Here's how the part is built. I have some questions about the finished solid (model axes, mm). Coordinates: 2 decimals unless noted, no trailing zeros. Write each loop counter-clockwise with the first axis right and the second up, starting at its lowest first coordinate (ties: lowest second). Pieces come first, ordered by that corner, then holes.
(1) Imagine slicing it at C-C, the plane y = 15. List the corners of the cut face in (x, z) for me, plus the area to 3 significant figures.
(2) Please list where these lines run through material, in increasing order: probe 1 along Y at (x, z) = (13, -1.2); probe 2 along Y at (x, z) = (128.5, -2.6); probe 3 along X at (y, z) = (39, -2.25).
(3) Imagine slicing it at A-A, the plane y = -23. List the corners of the cut face in (x, z) for me.
(4) Imagine slicing it at B-B, the plane x = 30. List the corners of the cut face in (y, z) for me, plus the area to 3 significant figures.
(5) Imagine slicing it at D-D, the plane z = -1.85. State how many separate pieces and enclosed holes the cut face has, plus the area to 3 significant figures.
```python
from build123d import *

# Parameters (mm, degrees)
SKETCH_1_W             = 270
SKETCH_1_H             = 150
SM_BASE_FLANGE_1_DEPTH = 4
FILLET_1_R             = 1
SKETCH_2_R             = 1.5
CUT_EXTRUDE_1_DEPTH    = 10
SKETCH_3_R             = 1.5
CUT_EXTRUDE_2_DEPTH    = 10
SKETCH_4_W             = 47
SKETCH_4_H             = 90
CUT_EXTRUDE_3_DEPTH    = 10
SKETCH_5_W             = 57
SKETCH_5_H             = 50
CUT_EXTRUDE_4_DEPTH    = 10
SKETCH_6_W             = 14
SKETCH_6_H             = 36.5
CUT_EXTRUDE_5_DEPTH    = 10


# Sheet-metal steps are written as plain solids
with BuildPart() as part:
    # Sketch 1 → 基体-法兰1 (new body)
    with BuildSketch(Plane.XY):
        Rectangle(SKETCH_1_W, SKETCH_1_H)
    extrude(amount=-SM_BASE_FLANGE_1_DEPTH)

    # 圆角1
    fillet_1_edges = [part.edges().sort_by_distance(p)[0] for p in [
        (135, -75, -2),
        (-135, -75, -2),
        (-135, 75, -2),
        (135, 75, -2),
    ]]
    fillet(fillet_1_edges, radius=FILLET_1_R)

    # Sketch 2 → 切除-拉伸1 (cut)
    with BuildSketch(Plane(origin=(0, 0, -4), x_dir=(-1, 0, 0), z_dir=(0, 0, -1))):
        with Locations((-13, -67.5)):
            Circle(SKETCH_2_R)
        with Locations((-13, -57.5)):
            Circle(SKETCH_2_R)
        with Locations((13, -57.5)):
            Circle(SKETCH_2_R)
        with Locations((13, -67.5)):
            Circle(SKETCH_2_R)
    extrude(amount=-CUT_EXTRUDE_1_DEPTH, mode=Mode.SUBTRACT)

    # 草图3 → 切除-拉伸2 (cut)
    with BuildSketch(Plane(origin=(0, 0, -4), x_dir=(-1, 0, 0), z_dir=(0, 0, -1))):
        with Locations((-128.5, 58)):
            Circle(SKETCH_3_R)
        with Locations((-128.5, 32)):
            Circle(SKETCH_3_R)
        with Locations((-118.5, 58)):
            Circle(SKETCH_3_R)
        with Locations((-118.5, 32)):
            Circle(SKETCH_3_R)
    cut_extrude_2 = extrude(amount=-CUT_EXTRUDE_2_DEPTH, mode=Mode.SUBTRACT)

    # 镜向1: 切除-拉伸2 across plane
    add(cut_extrude_2.mirror(Plane(origin=(0, 0, 0), x_dir=(0, 0, 1), z_dir=(1, 0, 0))), mode=Mode.SUBTRACT)

    # 草图4 → 切除-拉伸3 (cut)
    with BuildSketch(Plane(origin=(0, 0, -4), x_dir=(-1, 0, 0), z_dir=(0, 0, -1))):
        with Locations((-35, -2)):
            Rectangle(SKETCH_4_W, SKETCH_4_H)
    cut_extrude_3 = extrude(amount=-CUT_EXTRUDE_3_DEPTH, mode=Mode.SUBTRACT)

    # 草图5 → 切除-拉伸4 (cut)
    with BuildSketch(Plane.XY):
        with Locations((35, -4)):
            Rectangle(SKETCH_5_W, SKETCH_5_H)
    cut_extrude_4 = extrude(amount=-CUT_EXTRUDE_4_DEPTH, mode=Mode.SUBTRACT)

    # 草图6 → 切除-拉伸5 (cut)
    with BuildSketch(Plane.XY):
        with Locations((70.5, 2.75)):
            Rectangle(SKETCH_6_W, SKETCH_6_H)
    cut_extrude_5 = extrude(amount=-CUT_EXTRUDE_5_DEPTH, mode=Mode.SUBTRACT)

    # 镜向2: 切除-拉伸3, 切除-拉伸4, 切除-拉伸5 across plane
    add(cut_extrude_3.mirror(Plane(origin=(0, 0, 0), x_dir=(0, 0, 1), z_dir=(1, 0, 0))), mode=Mode.SUBTRACT)
    add(cut_extrude_4.mirror(Plane(origin=(0, 0, 0), x_dir=(0, 0, 1), z_dir=(1, 0, 0))), mode=Mode.SUBTRACT)
    add(cut_extrude_5.mirror(Plane(origin=(0, 0, 0), x_dir=(0, 0, 1), z_dir=(1, 0, 0))), mode=Mode.SUBTRACT)


solid = part.part
```
Recorded:
1. outline: (-135, -4) - (-77.5, -4) - (-77.5, 0) - (-135, 0) - close; (-6.5, -4) - (6.5, -4) - (6.5, 0) - (-6.5, 0) - close; (77.5, -4) - (135, -4) - (135, 0) - (77.5, 0) - close
1. area: 512 mm2
2. probe 1: y = -75 to -69, -66 to -59, -56 to -47, 43 to 75
2. probe 2: y = -75 to 30.5, 33.5 to 56.5, 59.5 to 75
2. probe 3: x = -135 to -58.5, -11.5 to 11.5, 58.5 to 135
3. outline: (-135, -4) - (-63.5, -4) - (-63.5, 0) - (-135, 0) - close; (-6.5, -4) - (6.5, -4) - (6.5, 0) - (-6.5, 0) - close; (63.5, -4) - (135, -4) - (135, 0) - (63.5, 0) - close
4. outline: (-75, -4) - (-47, -4) - (-47, 0) - (-75, 0) - close; (43, -4) - (75, -4) - (75, 0) - (43, 0) - close
4. area: 240 mm2
5. separate pieces: 1
5. enclosed holes: 14
5. area: 29,900 mm2
